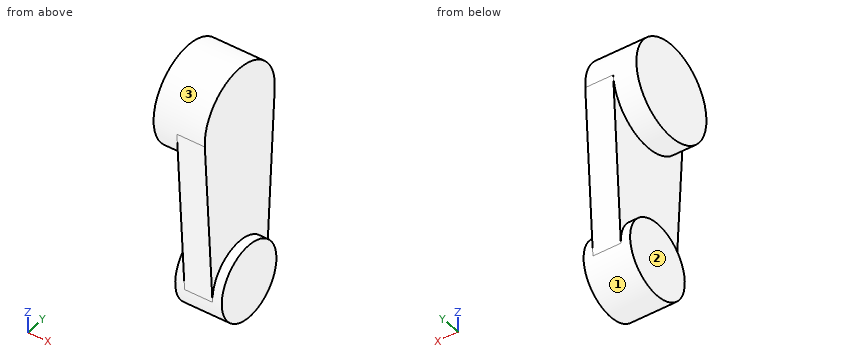
```python
from build123d import *
from build123d.topology import SkipClean

# Parameters (mm, degrees)
BOSS_EXTRUDE2_DEPTH      = 60
BOSS_EXTRUDE4_START      = 50
SKETCH5_R                = 102.5
BOSS_EXTRUDE4_DEPTH      = 50
BOSS_EXTRUDE7_DEPTH      = 20
BOSS_EXTRUDE7_DEPTH_BACK = 80
SKETCH6_R                = 80


with BuildPart() as part:
    # Sketch2 → Boss-Extrude2 (new body)
    with BuildSketch(Plane(origin=(0, 0, 0), x_dir=(0, 0, -1), z_dir=(1, 0, 0))):
        with BuildLine():
            Line((6.40625, 102.299608801), (365, 79.843597113))
            ThreePointArc((365, 79.843597113), (440, 0), (365, -79.843597113))
            Line((365, -79.843597113), (6.40625, -102.299608801))
            ThreePointArc((6.40625, -102.299608801), (-102.5, 0), (6.40625, 102.299608801))
        make_face()
    extrude(amount=BOSS_EXTRUDE2_DEPTH)

    # Sketch5 → Boss-Extrude4 (add)
    with BuildSketch(Plane.ZY.offset(BOSS_EXTRUDE4_START)):
        Circle(SKETCH5_R)
    extrude(amount=-BOSS_EXTRUDE4_DEPTH)

    # Sketch6 → Boss-Extrude7 (add, two sides: drawn at the far end of the back side and taken through both)
    with SkipClean():  # the faces are left unmerged after this step: merging them gives an invalid solid
        with BuildSketch(Plane.ZY.offset(-BOSS_EXTRUDE7_DEPTH_BACK)):
            with Locations((-360, 0)):
                Circle(SKETCH6_R)
        extrude(amount=BOSS_EXTRUDE7_DEPTH + BOSS_EXTRUDE7_DEPTH_BACK)


solid = part.part
```
The model under review builds one solid part; all positions refer to its coordinate system, in mm. Face numbers are marked on the shaded views. A direction names the side the tool comes from. Round coordinates to 2 decimals unless told otherwise and drop trailing zeros. Order: outer loops, then holes, each group sorted by start corner. A loop starts at its lowest first (then second) coordinate and runs counter-clockwise, first axis right, second up.
(1) For P1, Ø10, axis at x = -13, y = 52, coming from the -Z side; P2, Ø3, axis at x = 31, z = -298.5, coming from the +Y side; P3, Ø3, axis at x = 48.5, z = -316, coming from the -Y side, all flat-tipped, find the tip position at first contact; note any pin that passes through.
Working result:
P1: stops at z = -424.74
P2: stops at y = 84.1
P3: stops at y = -83.01
(2) Wall thickness on L1, parallel to X at y = -23.5, z = -185.5; L2, parallel to X at y = -75, z = -367.5; L3, parallel to Z at x = -36, y = -4.5: over which ranges is each line inside the solid? List them lowest first.
Working result:
L1: x = 0 to 60
L2: x = -20 to 80
L3: z = -102.4 to 102.4
(3) Tool access review of the marked faces 1, 2 and 3: name each direction out of +Z, -Z, +X, -X, +Y, -Y from which nothing blocks a thin tool from reaching the whole face with its end or side.
Working result:
face 1: none
face 2: -Z, -X, +Y, -Y
face 3: -X
(4) Take a section at B-B, the plane z = -360. State the section outline as (x, y) points.
Working result:
outline: (-20, -80) - (0, -80) - (0, -80.16) - (60, -80.16) - (60, -80) - (80, -80) - (80, 80) - (60, 80) - (60, 80.16) - (0, 80.16) - (0, 80) - (-20, 80) - close
(5) Take a section at D-D, the plane y = 67. State the section outline as (x, z) points.
Working result:
outline: (-50, -77.57) - (0, -77.57) - (0, -316.29) - (-20, -316.29) - (-20, -403.71) - (80, -403.71) - (80, -316.29) - (60, -316.29) - (60, 77.57) - (-50, 77.57) - close
(6) Take a section at C-C, the plane x = 16. State the section outline as (y, z) points.
Working result:
outline: (-102.3, -6.41) - (-79.84, -365) arc R80 ccw to (79.84, -365) - (102.3, -6.41) arc R102.5 ccw (long way) to start
(7) Take a section at A-A, the plane y = 38.5. State the section outline as (x, z) points, plus the area to 3 significant figures.
Working result:
outline: (-50, -94.99) - (0, -94.99) - (0, -289.87) - (-20, -289.87) - (-20, -430.13) - (80, -430.13) - (80, -289.87) - (60, -289.87) - (60, 94.99) - (-50, 94.99) - close
area: 46,600 mm2
